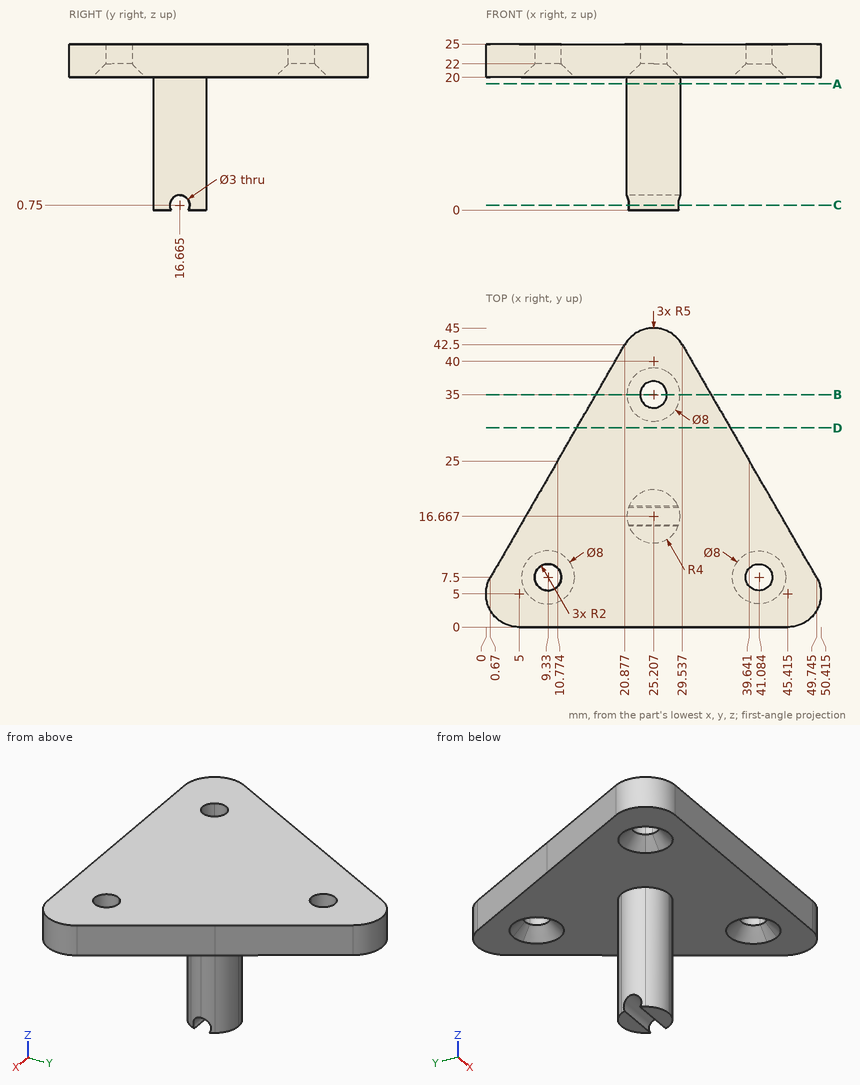
Check sheet for the drawn part. Datum: minimum x, y, z corner. Units: mm. Round coordinates to 2 decimals unless told otherwise and drop trailing zeros. Write each loop counter-clockwise with the first axis right and the second up, starting at its lowest first coordinate (ties: lowest second). Pieces come first, ordered by that corner, then holes. Notation, with made-up numbers: (83, 31) -> (89, 31) arc R29 cw to (89, 58) -> close; hole circle Ø11 at (-14.75, -14.5). An arc over 180 degrees is marked (long way). Write each question's results on one line, items separated by ' | '. Start each with the question number.
1. Material ranges on probe 1 along X at (y, z) = (7, 21.75) (1 decimal); probe 2 along Z at (x, y) = (29, 8); probe 3 along Y at (x, z) = (25.5, 17.5) (1 decimal), recorded low to high. Write a range as from..to.
2. Cross-section at C-C (z = 0.75). Enter the section's corners in (x, y) (1 decimal).
3. Depth check by flat-ended pin: P1, Ø1, axis at x = 23, z = 22, coming from the +Y side; P2, Ø10, axis at x = 13, z = 13, coming from the +Y side; P3, Ø8, axis at y = 15, z = 8.5, coming from the -X side; P4, Ø6, axis at y = 39.5, z = 21, coming from the -X side. Enter the tip coordinate at first touch or a pass-through.
4. Cross-section at B-B (y = 35). Enter the section's corners in (x, z).
5. Cross-section at A-A (z = 19). Enter the section's corners in (x, y).
6. Cross-section at D-D (y = 30). Enter the section's corners in (x, z) (1 decimal).
Solutions:
1) probe 1: x = 0.4..7.1, 11.5..38.9, 43.3..50 | probe 2: z = 20..25 | probe 3: y = 12.7..20.7
2) outline: (21.5, 15.2) arc R4 ccw to (28.9, 15.2) -> close; (21.5, 18.2) -> (28.9, 18.2) arc R4 ccw to start
3) P1: stops at y = 44.7 | P2: passes through | P3: stops at x = 21.21 | P4: stops at x = 17.41
4) outline: (16.55, 20) -> (21.21, 20) -> (23.21, 22) -> (23.21, 25) -> (16.55, 25) -> close; (27.21, 22) -> (29.21, 20) -> (33.87, 20) -> (33.87, 25) -> (27.21, 25) -> close
5) outline: circle Ø8 at (25.21, 16.67)
6) outline: (13.7, 20) -> (36.8, 20) -> (36.8, 25) -> (13.7, 25) -> close
